Design review of the part shown in the three views and the two pictorial views. Dimensions are in mm from the part's minimum x, y and z. A direction names the side the tool comes from. Coordinates: 2 decimals unless noted, no trailing zeros. Order: outer loops, then holes, each group sorted by start corner. A loop starts at its lowest first (then second) coordinate and runs counter-clockwise, first axis right, second up. Notation, with made-up numbers: (40, 15) -> (88, 15) arc R18 cw to (88, 32) -> close; hole circle Ø9 at (75, 69). An arc over 180 degrees is marked (long way). Answer as a JSON object with one key per item and string values. Group by question number.
1) For pin 1 (17 mm diameter, centred on x = 96, y = 70, fed in from +Z); pin 2 (2 mm diameter, centred on y = 126.5, z = 7, fed in from -X); pin 3 (12 mm diameter, centred on y = 95, z = 22, fed in from +X); pin 4 (10 mm diameter, centred on x = 96.5, y = 107, fed in from +Z) (1 decimal), all flat-tipped, find the tip position at first contact; note any pin that passes through.
2) Wall thickness on L1, parallel to Z at x = 24, y = 80; L2, parallel to Y at x = 69, z = 27.5 (1 decimal); L3, parallel to Z at x = 88, y = 109 (1 decimal): over which ranges is each line inside the solid? List them lowest first.
3) Machinability: for the marked faces 1 and 2, which of the approach directions +Z, -Z, +X, -X, +Y, -Y give a long, thin tool a straight path to every point of the face, cutting with its end or side? Answer none if there is none.
4) Add section A-A, the plane x = 59.5. Write out the cut boundary in (y, z) (1 decimal).
5) Add section B-B, the plane y = 90.5. Write out the cut boundary in (x, z).
6) Add section C-C, the plane z = 17. Write out the cut boundary in (x, y), then the cut area to 3 significant figures.
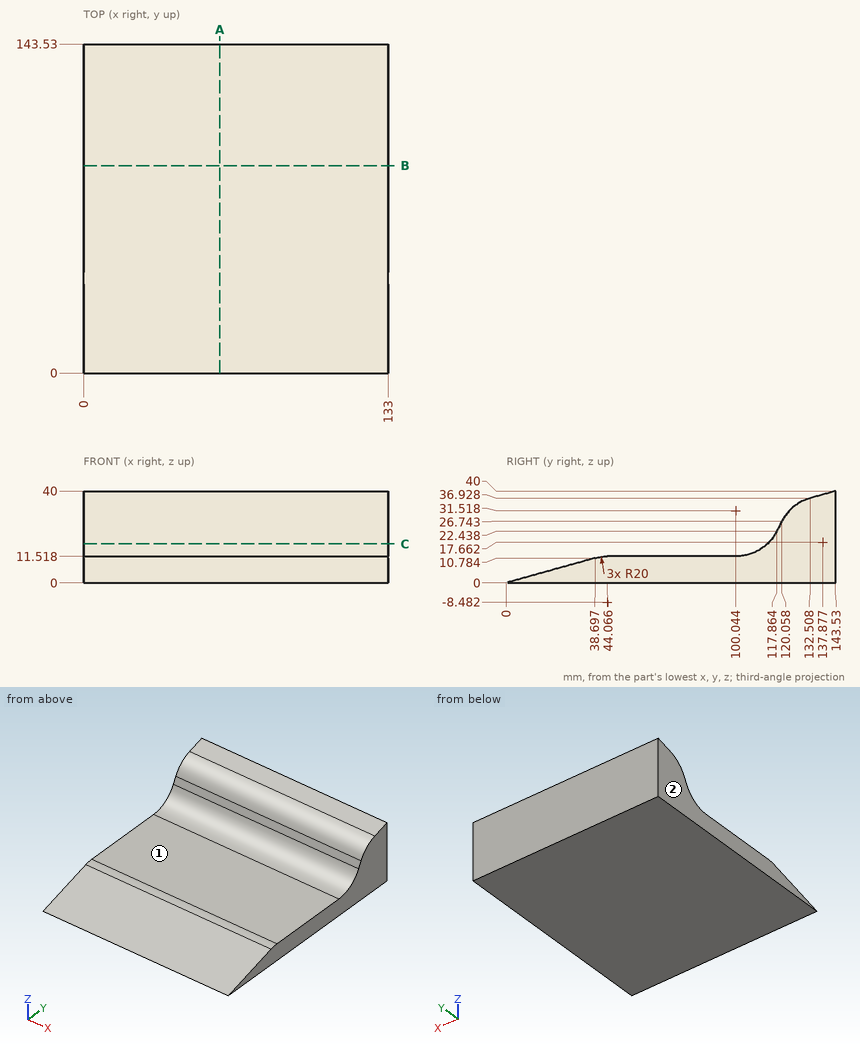
Output values:
{
 "1": {"pin 1": "stops at z = 11.52", "pin 2": "stops at x = 0", "pin 3": "passes through", "pin 4": "stops at z = 15.5"},
 "2": {"L1": "z = 0 to 11.52", "L2": "y = 120.5 to 143.5", "L3": "z = 0 to 13.6"},
 "3": {"face 1": "+Z, +X, -X, -Y", "face 2": "+Z, -Z, -X, +Y, -Y"},
 "4": {"outline": "(0, 0) -> (143.5, 0) -> (143.5, 40) -> (132.5, 36.9) arc R20 ccw to (120.1, 26.7) -> (117.9, 22.4) arc R20 cw to (100, 11.5) -> (44.1, 11.5) arc R20 ccw to (38.7, 10.8) -> close"},
 "5": {"outline": "(0, 0) -> (133, 0) -> (133, 11.52) -> (0, 11.52) -> close"},
 "6": {"outline": "(0, 113.8) -> (133, 113.8) -> (133, 143.53) -> (0, 143.53) -> close", "area": "3,950 mm²"}
}
